Design review of the part built by this model. Coordinates are the model's own, in mm. Face numbers are marked on the shaded views. A direction names the side the tool comes from. Give positions to 0.01 mm unless a question says otherwise; leave off trailing zeros. Order: outer loops, then holes, each group sorted by start corner. A loop starts at its lowest first (then second) coordinate and runs counter-clockwise, first axis right, second up. Notation, with made-up numbers: (15, 30.5) -> (53, 30.5) arc R24 ccw to (53, 69.5) -> close; hole circle Ø5 at (87.5, 63). An arc over 180 degrees is marked (long way). One line per item, written item: value. Start each with the question number.
1) Wall thickness on line 1 along Y through (x, z) = (0, 2.5); line 2 along Y through (x, z) = (-18, -17.5); line 3 along Z through (x, y) = (-7, -1.5): over which ranges is each line inside the solid? List them lowest first. Write a range as from..to.
2) Consider section D-D (z = -17.5). State the section outline as (x, y) points, plus the area to 3 significant figures.
3) For pin 1 (20 mm diameter, centred on x = -5, y = 0, fed in from -Z); pin 2 (2 mm diameter, centred on x = 8.5, y = -23.5, fed in from +Z); pin 3 (7 mm diameter, centred on y = -12, z = 3, fed in from -X), all flat-tipped, find the tip position at first contact; note any pin that passes through.
4) Consider section C-C (y = -7). State the section outline as (x, z) points.
5) Tool access review of the marked faces 1, 2, 3 and 4: name each direction out of +Z, -Z, +X, -X, +Y, -Y from which nothing blocks a thin tool from reaching the whole face with its end or side.
6) Consider section B-B (x = 0). State the section outline as (y, z) points.
7) Consider section A-A (z = 5). State the section outline as (x, y) points.
Autodesk Inventor part; units mm, degrees
ref_plane "YZ Plane" through (0, 0, 0) normal (1, 0, 0) x (0, 1, 0)
ref_plane "XZ Plane" through (0, 0, 0) normal (0, 1, 0) x (-1, 0, 0)
ref_plane "XY Plane" through (0, 0, 0) normal (0, 0, 1) x (1, 0, 0)
sketch "Sketch1" plane through (0, 0, 0) normal (0, 0, 1) x (1, 0, 0)
  circle A0 centre (0, 0) radius 35
  line L0 (-35, 0) -> (-35, -40)
  line L1 (-35, -40) -> (35, -40)
  line L2 (35, -40) -> (35, 0)
  dimension "d0" = 70
  dimension "d1" = 40
extrude "Extrusion1" add sketch "Sketch1" along normal blind 12.5
sketch "Sketch2" plane through (-35, -40, 0) normal (0, -1, 0) x (1, 0, 0)
  arc A0 (82.5, -22.5) -> (-12.5, -22.5) centre (35, -22.5) ccw
  line L0 (0, 12.5) -> (70, 12.5) construction
  line L1 (35, 12.5) -> (35, 0)
  line L2 (82.5, -22.5) -> (-12.5, -22.5)
  arc A1 (-12.5, -22.5) -> (82.5, -22.5) centre (35, -22.5) ccw construction
  dimension "d4" = 95
  dimension "d6" = 35
extrude "Extrusion2" add sketch "Sketch2" along normal blind 8
chamfer "Chamfer1" distance 3.5 angle 45 3 edges at (0, 35, 12.5) (-35, -20, 12.5) (35, -20, 12.5)
sketch "Sketch3" plane through (0, 0, 0) normal (0, 0, -1) x (-1, 0, 0)
  circle A0 centre (0, 0) radius 12.5
  dimension "d12" = 25
extrude "Extrusion3" cut sketch "Sketch3" against normal blind 7
sketch "Sketch4" plane through (-35, -48, 0) normal (0, -1, 0) x (1, 0, 0)
  arc A0 (82.5, -22.5) -> (-12.5, -22.5) centre (35, -22.5) ccw
  arc A1 (77.5, -22.5) -> (-7.5, -22.5) centre (35, -22.5) ccw
  arc A2 (82.5, -22.5) -> (-12.5, -22.5) centre (35, -22.5) ccw
  line L0 (-7.5, -22.5) -> (-12.5, -22.5)
  line L1 (82.5, -22.5) -> (77.5, -22.5)
  line L2 (-12.5, -22.5) -> (82.5, -22.5)
  circle A3 centre (35, -22.5) radius 32.5
  circle A4 centre (35, -22.5) radius 30
  point P0 (35, 0)
  point P1 (5, -22.5)
  point P2 (65, -22.5)
  point P3 (67.5, -22.5)
  point P4 (2.5, -22.5)
  dimension "d16" = 5
  dimension "d20" = 65
  dimension "d21" = 60
extrude "Extrusion4" cut sketch "Sketch4" against normal blind 4 contours L1 A1 L0 A0 | L2 A4 A3 picked at (43.6934, 7.7339)
properties part number "Base 1 left"
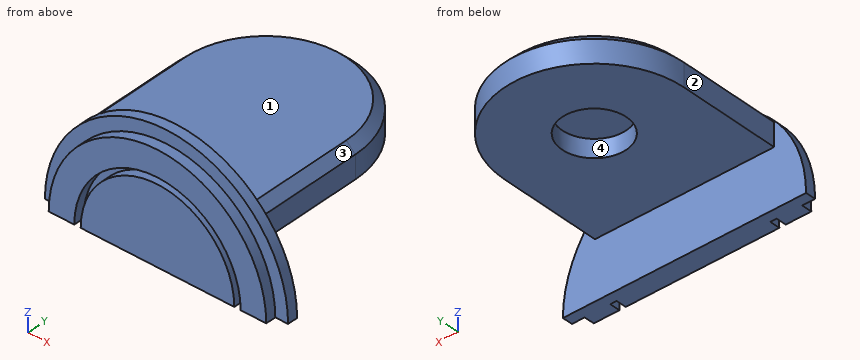
Checked values:
1. line 1: y = -48..-12.5, 12.5..35
1. line 2: y = -48..-40
1. line 3: z = 7..12.5
2. outline: (-47.24, -44) -> (-42.2, -44) -> (-42.2, -48) -> (-32.11, -48) -> (-32.11, -44) -> (-29.58, -44) -> (-29.58, -48) -> (29.58, -48) -> (29.58, -44) -> (32.11, -44) -> (32.11, -48) -> (42.2, -48) -> (42.2, -44) -> (47.24, -44) -> (47.24, -40) -> (-47.24, -40) -> close
2. area: 695 mm^2
3. pin 1: stops at z = 0
3. pin 2: stops at z = 12.5
3. pin 3: stops at x = -35
4. outline: (-35, 0) -> (-10.36, 0) -> (-10.36, 7) -> (10.36, 7) -> (10.36, 0) -> (35, 0) -> (35, 9) -> (31.5, 12.5) -> (-31.5, 12.5) -> (-35, 9) -> close
5. face 1: +Z, +X, -X, +Y
5. face 2: +Z, -Z, -X, +Y
5. face 3: +Z, +X, +Y
5. face 4: -Z
6. outline: (-48, -22.5) -> (-40, -22.5) -> (-40, 0) -> (-12.5, 0) -> (-12.5, 7) -> (12.5, 7) -> (12.5, 0) -> (35, 0) -> (35, 9) -> (31.5, 12.5) -> (-40, 12.5) -> (-40, 25) -> (-44, 25) -> (-44, 20) -> (-48, 20) -> (-48, 10) -> (-44, 10) -> (-44, 7.5) -> (-48, 7.5) -> close
7. outline: (-38.73, -44) -> (-32.4, -44) -> (-32.4, -48) -> (-17.32, -48) -> (-17.32, -44) -> (-11.99, -44) -> (-11.99, -48) -> (11.99, -48) -> (11.99, -44) -> (17.32, -44) -> (17.32, -48) -> (32.4, -48) -> (32.4, -44) -> (38.73, -44) -> (38.73, -40) -> (35, -40) -> (35, 0) arc R35 ccw to (-35, 0) -> (-35, -40) -> (-38.73, -40) -> close; hole circle Ø25 at (0, 0)
